```python
from build123d import *

# Parameters (mm, degrees)
SKETCH2_W           = 304.8
SKETCH2_H           = 609.6
BOSS_EXTRUDE1_DEPTH = 5
SKETCH3_W           = 10
SKETCH3_H           = 610
EXTRUDE_THIN1_DEPTH = 2.5
SKETCH4_W           = 10
SKETCH4_H           = 610
EXTRUDE_THIN2_DEPTH = 2.5
BOSS_EXTRUDE2_DEPTH = 5
EXTRUDE_THIN3_DEPTH = 4
EXTRUDE_THIN5_DEPTH = 5
SKETCH12_W          = 309.8
SKETCH12_H          = 215.656941329
CUT_EXTRUDE1_DEPTH  = 615


with BuildPart() as part:
    # Sketch2 → Boss-Extrude1 (new body)
    with BuildSketch(Plane(origin=(0, 0, 0), x_dir=(1, 0, 0), z_dir=(0, 1, 0))):
        Rectangle(SKETCH2_W, SKETCH2_H)
    extrude(amount=BOSS_EXTRUDE1_DEPTH)

    # Sketch3 → Extrude-Thin1 (add, symmetric)
    with BuildSketch(Plane(origin=(152.4, 0, 0), x_dir=(0, 0, -1), z_dir=(1, 0, 0))):
        with Locations((-304.8, 310)):
            Rectangle(SKETCH3_W, SKETCH3_H)
        with Locations((304.8, 310)):
            Rectangle(SKETCH3_W, SKETCH3_H)
    extrude(amount=EXTRUDE_THIN1_DEPTH, both=True)

    # Sketch4 → Extrude-Thin2 (add, symmetric)
    with BuildSketch(Plane.ZY.offset(152.4)):
        with Locations((-304.8, 310)):
            Rectangle(SKETCH4_W, SKETCH4_H)
        with Locations((304.8, 310)):
            Rectangle(SKETCH4_W, SKETCH4_H)
    extrude(amount=EXTRUDE_THIN2_DEPTH, both=True)

    # Sketch5 → Boss-Extrude2 (add)
    with BuildSketch(Plane(origin=(0, 615, 0), x_dir=(1, 0, 0), z_dir=(0, 1, 0))):
        Polygon((154.9, -309.8), (-154.9, -309.8), (-154.9, -299.8), (-5, -299.8), (-5, -99.8), (-5, -91.133474836), (-187, 224.099772141), (-154.9, 309.8), (-149.9, 309.8), (-149.9, 224.099772141), (149.9, 224.099772141), (149.9, 309.8), (154.9, 309.8), (187, 224.099772141), (5, -91.133474836), (5, -104.787457748), (5, -299.8), (154.9, -299.8), align=None)
    extrude(amount=BOSS_EXTRUDE2_DEPTH)

    # Sketch6 → Extrude-Thin3 (add)
    with BuildSketch(Plane.ZY.offset(154.9)):
        Polygon((-224.099772141, 615), (-299.8, 565), (-302.555663937, 569.172087759), (-226.855436078, 619.172087759), align=None)
    extrude(amount=-EXTRUDE_THIN3_DEPTH)

    # Sketch11 → Extrude-Thin5 (add)
    with BuildSketch(Plane(origin=(154.9, 0, 0), x_dir=(0, 0, -1), z_dir=(1, 0, 0))):
        Polygon((224.099772141, 620), (309.8, 565), (307.099444062, 560.792031651), (221.399216204, 615.792031651), align=None)
    extrude(amount=-EXTRUDE_THIN5_DEPTH)

    # Sketch12 → Cut-Extrude1 (cut)
    with BuildSketch(Plane(origin=(0, 620, 0), x_dir=(1, 0, 0), z_dir=(0, 1, 0))):
        with Locations((0, -201.971529336)):
            Rectangle(SKETCH12_W, SKETCH12_H)
    extrude(amount=-CUT_EXTRUDE1_DEPTH, mode=Mode.SUBTRACT)


solid = part.part
```
Check sheet for the modelled part. Datum: model origin and axes. Units: mm. A direction names the side the tool comes from. Give positions to 0.01 mm unless a question says otherwise; leave off trailing zeros. Write each loop counter-clockwise with the first axis right and the second up, starting at its lowest first coordinate (ties: lowest second). Pieces come first, ordered by that corner, then holes. Notation, with made-up numbers: (42.5, 56.25) - (96.5, 56.25) arc R21 ccw to (96.5, 92.25) - close; hole circle Ø4 at (45, -23). An arc over 180 degrees is marked (long way). Answer as a JSON object with one key per item and string values. Group by question number.
1) Sectioned sample at D-D (z = 250.5). Record the cut outline in (x, y).
2) Depth check by flat-ended pin: P1, Ø1.5, axis at x = -151.5, z = -305.5, coming from the -Y side; P2, Ø4, axis at x = 130, z = 111, coming from the +Y side; P3, Ø5.5, axis at x = -151.5, y = 370.5, coming from the +Z side; P4, Ø1.5, axis at x = -25.5, y = 2.5, coming from the -Z side. Enter the tip coordinate at first touch or a pass-through.
3) Thickness scan on probe 1 along Y at (x, z) = (-110, -209); probe 2 along Y at (x, z) = (-40.5, 50); probe 3 along Y at (x, z) = (165, -194). Record the ranges inside material, lowest first. Write a range as from..to.
4) Sectioned sample at B-B (x = -125). Record the cut outline in (y, z).
5) Sectioned sample at C-C (z = -242). Record the cut outline in (x, y).
6) Sectioned sample at A-A (y = 135). Record the cut outline in (x, z), then the cut area to 3 significant figures.
7) Release check for a two-part mould opening along Y. For faces 1 (the face through (-2, 0, -4)), 2 (the face through (-154.9, 334, -302)), 3 (the face through (-152.93, 590.35, -261.42)), 4 (the face through (152.435, 593.514, -265.37)) record: pulls with the +Y half, pulls with the -Y half, needs draft (parallel to the pull), parting line crosses it, or undercut.
8) Access from +Z, -Z, +X, -X, +Y, -Y to the whole of each face (thin tool, end or side, straight path). Record for faces 5 (the face through (154.9, 334, -302)), 6 (the face through (97.274, 617.465, -68.69)), 7 (the face through (-94.73, 617.46, -64.28)).
Geometry results:
{
 "1": {"outline": "(-152.4, 0) - (152.4, 0) - (152.4, 5) - (-152.4, 5) - close"},
 "2": {"P1": "stops at y = 0", "P2": "stops at y = 5", "P3": "stops at z = -299.8", "P4": "stops at z = -304.8"},
 "3": {"probe 1": "y = 0..5, 615..620", "probe 2": "y = 0..5", "probe 3": "y = 615..620"},
 "4": {"outline": "(0, -304.8) - (5, -304.8) - (5, 304.8) - (0, 304.8) - close; (615, -224.1) - (620, -224.1) - (620, -116.71) - (615, -116.71) - close"},
 "5": {"outline": "(-180.3, 615) - (-149.9, 615) - (-149.9, 620) - (-180.3, 620) - close; (-154.9, 603.18) - (-150.9, 603.18) - (-150.9, 609.17) - (-154.9, 609.17) - close; (-152.4, 0) - (152.4, 0) - (152.4, 5) - (-152.4, 5) - close; (149.9, 602.57) - (154.9, 602.57) - (154.9, 608.51) - (149.9, 608.51) - close; (149.9, 615) - (180.3, 615) - (180.3, 620) - (149.9, 620) - close"},
 "6": {"outline": "(-154.9, -309.8) - (-149.9, -309.8) - (-149.9, -299.8) - (-154.9, -299.8) - close; (149.9, -309.8) - (154.9, -309.8) - (154.9, -299.8) - (149.9, -299.8) - close", "area": "100 mm^2"},
 "7": {"face 1": "pulls with the -Y half", "face 2": "needs draft", "face 3": "undercut", "face 4": "undercut"},
 "8": {"face 5": "+Z, -Z, +X, -Y", "face 6": "+Z, +X, +Y", "face 7": "+Z, -X, +Y"}
}
